Read the model definition and answer for the solid it produces. Units are mm, in the model's axes. Face numbers are marked on the shaded views. Round coordinates to 2 decimals unless told otherwise and drop trailing zeros. Write each loop counter-clockwise with the first axis right and the second up, starting at its lowest first coordinate (ties: lowest second). Pieces come first, ordered by that corner, then holes. Notation, with made-up numbers: M 64.25,-7.75 L 101.25,-7.75 A26 cw 101.25,14.25 Z; hole C -25.5,9.25 d6. An arc over 180 degrees is marked long. Use one line per item in the form item = value. Start each with the question number.
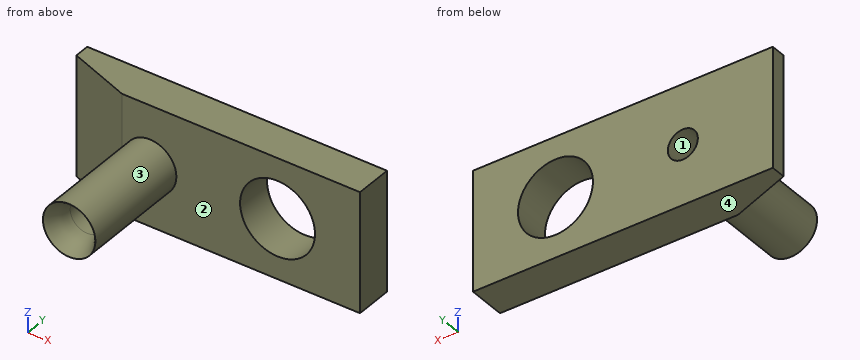
```python
from build123d import *

# Parameters (mm, degrees)
F0_R     = 5
F1_DEPTH = 5
F2_R     = 3.5
F2_R_2   = 2.25
F3_DEPTH = 15
F5_SIZE2 = 8.2424322584
F5_SIZE  = 3


# Not quite as in the source:
# - a fillet or chamfer that OpenCascade refuses, or shapes differently, is made with other operations: its cross-section is extruded or revolved along the edge and cut away or added


with BuildPart() as f1:
    # F0 (on Front) → F1 (new body)
    with BuildSketch(Plane.XZ):
        Polygon((-20, -8), (20, -8), (20, 0), (20, 8), (-20, 8), (-20, 0), align=None)
        with BuildLine():
            ThreePointArc((-6, 0), (-8, -2), (-10, 0))
            ThreePointArc((-10, 0), (-8, 2), (-6, 0))
        make_face(mode=Mode.SUBTRACT)
        with Locations((9, 0)):
            Circle(F0_R, mode=Mode.SUBTRACT)
    extrude(amount=F1_DEPTH)

    # F2 (on face) → F3 (join)
    with BuildSketch(Plane.XZ.offset(5)):
        with Locations((-8, 0)):
            Circle(F2_R)
        with Locations((-8, 0)):
            Circle(F2_R_2, mode=Mode.SUBTRACT)
    extrude(amount=F3_DEPTH)

    # F4: fillet of radius 5 on 1 edges, made by hand

    # F4_s1 → F4_t2 (revolve, cut)
    with BuildSketch(Plane.XY):
        with BuildLine():
            ThreePointArc((-4.5, -20), (-5.4270717335, -18.4605778141), (-5.75, -16.6928108612))
            Line((-5.75, -16.6928108612), (-5.75, -20))
            Line((-5.75, -20), (-4.5, -20))
        make_face()
    revolve(axis=Axis((-8, -20, 0), (0, -1, 0)), mode=Mode.SUBTRACT)

    # F5
    f5_edges = [f1.edges().sort_by_distance(p)[0] for p in [
        (-20, -5, 0),
    ]]
    f5_side = f1.faces().sort_by_distance((-20, -2.5, 0))[0]
    chamfer(f5_edges, length=F5_SIZE, length2=F5_SIZE2, reference=f5_side)


solid = f1.part
```
Q1. Each of these flat-tipped pins is pushed along its axis until it touches: pin 1 Ø1 at (y, z) = (-14, 2.5) entering from -X; pin 2 Ø6 at (y, z) = (-15, 2.5) entering from -X; pin 3 Ø4 at (y, z) = (-17.5, -3.5) entering from +X. Where does it stop, or does it pass through?
Q2. Find section B-B on x = 9. Write down the section's boundary in (y, z).
Q3. Find section C-C on x = -8. Write down the section's boundary in (y, z).
Q4. Find section A-A on z = 0. Write down the section's boundary in (x, y).
Q5. Find section D-D on z = 6. Write down the section's boundary in (x, y).
Q6. For a pull along Z with two mould halves and no side action, classify the marked faces 1, 2, 3 and 4 as +Z half, -Z half, draft (parallel to the pull), parting line (faces both ways), or undercut.
Q7. Straight lines are drawn through the part: line 1 (Z direction, x = -8, y = -1); line 2 (Z direction, x = -8, y = -13); line 3 (Y direction, x = -5.5, z = 2.75). For each, find the intervals that lie inside material, in ascending order. Write a range as [from, to].
Response:
q1.pin_1 = -10.87
q1.pin_2 = -11.5
q1.pin_3 = -4.84
q2.outline = M -5,-8 L 0,-8 L 0,-5 L -5,-5 Z; M -5,5 L 0,5 L 0,8 L -5,8 Z
q3.outline = M -20,-3.5 L -5,-3.5 L -5,-8 L 0,-8 L 0,-2 L -5,-2 L -5,-2.25 L -16.69,-2.25 A5 ccw Z; M -20,3.5 A5 ccw -16.69,2.25 L -5,2.25 L -5,2 L 0,2 L 0,8 L -5,8 L -5,3.5 Z
q4.outline = M -20,-2 L -11.76,-5 L -11.5,-5 L -11.5,-20 A5 ccw -10.25,-16.69 L -10.25,-5 L -10,-5 L -10,0 L -20,0 Z; M -6,-5 L -5.75,-5 L -5.75,-16.69 A5 ccw -4.5,-20 L -4.5,-5 L 4,-5 L 4,0 L -6,0 Z; M 14,-5 L 20,-5 L 20,0 L 14,0 Z
q5.outline = M -20,-2 L -11.76,-5 L 20,-5 L 20,0 L -20,0 Z
q6.face_1 = undercut
q6.face_2 = draft
q6.face_3 = parting line
q6.face_4 = -Z half
q7.line_1 = [-8, -2], [2, 8]
q7.line_2 = [-3.5, -2.25], [2.25, 3.5]
q7.line_3 = [-5, 0]
